```python
from build123d import *

# Parameters (mm, degrees)
F1_DEPTH  = 25.4
F2_R      = 3.175
F4_DEPTH  = 32.386
F5_R      = 6.35
F6_W      = 70.612
F6_H      = 12.7
F7_DEPTH  = 3.175
F8_R      = 3.175
F9_W      = 22.86
F9_H      = 3.175
F10_DEPTH = 25.4
F11_R     = 1.524


with BuildPart() as f1:
    # F0 (on Top) → F1 (new body)
    with BuildSketch(Plane.XY):
        Polygon((-35.306, 29.21), (0, 29.21), (35.306, 29.21), (35.306, 0), (63.881, 0), (63.881, 3.175), (38.481, 3.175), (38.481, 32.385), (0, 32.385), (-38.481, 32.385), (-38.481, 3.175), (-63.881, 3.175), (-63.881, 0), (-35.306, 0), align=None)
    extrude(amount=F1_DEPTH)

    # F2
    f2_edges = [f1.edges().sort_by_distance(p)[0] for p in [
        (-35.306, 0, 12.7),
        (35.306, 0, 12.7),
    ]]
    fillet(f2_edges, radius=F2_R)

    # F3 (on Front) → F4 (cut, through all)
    with BuildSketch(Plane.XZ):
        with BuildLine():
            ThreePointArc((-53.594, 7.8105), (-51.181, 5.3975), (-48.768, 7.8105))
            Line((-48.768, 7.8105), (-48.768, 17.4625))
            ThreePointArc((-48.768, 17.4625), (-51.181, 19.8755), (-53.594, 17.4625))
            Line((-53.594, 17.4625), (-53.594, 7.8105))
        make_face()
        with BuildLine():
            ThreePointArc((53.594, 17.4498), (51.181, 19.8628), (48.768, 17.4498))
            Line((48.768, 17.4498), (48.768, 7.7978))
            ThreePointArc((48.768, 7.7978), (51.181, 5.3848), (53.594, 7.7978))
            Line((53.594, 7.7978), (53.594, 17.4498))
        make_face()
    extrude(amount=-F4_DEPTH, mode=Mode.SUBTRACT)

    # F5
    f5_edges = [f1.edges().sort_by_distance(p)[0] for p in [
        (-63.881, 1.5875, 0),
        (-63.881, 1.5875, 25.4),
        (63.881, 1.5875, 25.4),
        (63.881, 1.5875, 0),
    ]]
    fillet(f5_edges, radius=F5_R)

    # F6 (on face) → F7 (join)
    with BuildSketch(Plane(origin=(0, 0, 0), x_dir=(1, 0, 0), z_dir=(0, 0, -1))):
        with Locations((0, -22.86)):
            Rectangle(F6_W, F6_H)
    extrude(amount=-F7_DEPTH)

    # F8
    f8_edges = [f1.edges().sort_by_distance(p)[0] for p in [
        (38.481, 3.175, 12.7),
        (38.481, 32.385, 12.7),
        (-38.481, 32.385, 12.7),
        (-38.481, 3.175, 12.7),
        (35.306, 16.51, 1.5875),
        (-35.306, 16.51, 1.5875),
    ]]
    fillet(f8_edges, radius=F8_R)

    # F9 (on face) → F10 (cut)
    with BuildSketch(Plane.XY.offset(3.175)):
        with Locations((0, 18.0975)):
            Rectangle(F9_W, F9_H)
    extrude(amount=-F10_DEPTH, mode=Mode.SUBTRACT)

    # F11
    f11_edges = [f1.edges().sort_by_distance(p)[0] for p in [
        (-11.43, 16.51, 1.5875),
        (11.43, 16.51, 1.5875),
    ]]
    fillet(f11_edges, radius=F11_R)


solid = f1.part
```
Input: part model. Units: mm. Frame: model coordinates. A direction names the side the tool comes from. Round coordinates to 2 decimals unless told otherwise and drop trailing zeros. Loops run counter-clockwise (first coordinate to the right, second up) from the corner with the lowest first, then second, coordinate; pieces in that order, holes last. Notation, with made-up numbers: (-36, 5.25) -> (-26, 5.25) arc R28 ccw to (-26, 36.25) -> close; hole circle Ø8 at (78.5, 1). An arc over 180 degrees is marked (long way). One line per item, written item: value.
(1) Section B-B (y = 14.5). Return the cut outline in (x, z) (3 decimals), plus the area to 3 significant figures.
Geometry check:
outline: (-38.481, 0) -> (-35.085, 0) -> (-35.085, 3.175) -> (-35.306, 3.175) -> (-35.306, 25.4) -> (-38.481, 25.4) -> close; (35.085, 0) -> (38.481, 0) -> (38.481, 25.4) -> (35.306, 25.4) -> (35.306, 3.175) -> (35.085, 3.175) -> close
area: 163 mm2
(2) Mould query, pull axis X, two halves, no side actions, for faces 1 (the face through (38.481, 18, 13)), 2 (the face through (0, 23, 3.175)), 3 (the face through (-37.526, 31.48, 12.878)). Classes: pulls with the +X half, pulls with the -X half, needs draft (parallel to the pull), parting line crosses it, or undercut.
Geometry check:
face 1: pulls with the +X half
face 2: undercut
face 3: pulls with the -X half
(3) Material intervals for line 1 (X direction, y = 20, z = 18.75); line 2 (Y direction, x = -17, z = 7) (3 decimals); line 3 (X direction, y = 2, z = 21.25), sorted ascending. Write a range as [from, to].
Geometry check:
line 1: [-38.48, -35.31], [35.31, 38.48]
line 2: [29.21, 32.385]
line 3: [-63.49, -35.53], [35.53, 63.49]
(4) Pin query (flat end, axial travel): pin 1 (12.5 mm diameter, centred on x = 14.5, y = 20.5, fed in from +Z) (3 decimals); pin 2 (11 mm diameter, centred on x = 1.5, z = 18, fed in from -Y); pin 3 (1.5 mm diameter, centred on y = 26.5, z = 10, fed in from -X); pin 4 (8 mm diameter, centred on x = -10.5, y = 27, fed in from -Z). Return the tip coordinate at first contact, or that it passes through.
Geometry check:
pin 1: z = 3.175
pin 2: y = 29.21
pin 3: x = -38.48
pin 4: z = 0
(5) Section C-C (x = 7.5). Return the cut outline in (y, z) (3 decimals), plus the area to 3 significant figures.
Geometry check:
outline: (19.685, 0) -> (32.385, 0) -> (32.385, 25.4) -> (29.21, 25.4) -> (29.21, 3.175) -> (19.685, 3.175) -> close
area: 111 mm2
(6) Set-up query: faces 4 (the face through (-34.351, 15.605, 1.61)), 5 (the face through (51.128, 1.565, 5.385)), 6 (the face through (55, 3.175, 13)). Return all of +Z, -Z, +X, -X, +Y, -Y with unobstructed straight access to the full face (end or side cutting, diameter ignored); none if empty.
Geometry check:
face 4: +Z, -Z, -Y
face 5: +Y, -Y
face 6: +Z, -Z, +X, +Y
(7) Section A-A (z = 16.25). Return the cut outline in (x, y) (3 decimals).
Geometry check:
outline: (-63.881, 0) -> (-53.594, 0) -> (-53.594, 3.175) -> (-63.881, 3.175) -> close; (-48.768, 0) -> (-38.481, 0) arc R3.175 ccw to (-35.306, 3.175) -> (-35.306, 29.21) -> (35.306, 29.21) -> (35.306, 3.175) arc R3.175 ccw to (38.481, 0) -> (48.768, 0) -> (48.768, 3.175) -> (41.656, 3.175) arc R3.175 cw to (38.481, 6.35) -> (38.481, 29.21) arc R3.175 ccw to (35.306, 32.385) -> (-35.306, 32.385) arc R3.175 ccw to (-38.481, 29.21) -> (-38.481, 6.35) arc R3.175 cw to (-41.656, 3.175) -> (-48.768, 3.175) -> close; (53.594, 0) -> (63.881, 0) -> (63.881, 3.175) -> (53.594, 3.175) -> close
(8) Section D-D (y = 22.5). Return the cut outline in (x, z) (3 decimals).
Geometry check:
outline: (-38.481, 0) -> (38.481, 0) -> (38.481, 25.4) -> (35.306, 25.4) -> (35.306, 3.175) -> (-35.306, 3.175) -> (-35.306, 25.4) -> (-38.481, 25.4) -> close
